Geometry check sheet. Reference: the model listing, model coordinates, mm. Face numbers are marked on the shaded views. A direction names the side the tool comes from. Give positions to 0.01 mm unless a question says otherwise; leave off trailing zeros. Loops run counter-clockwise (first coordinate to the right, second up) from the corner with the lowest first, then second, coordinate; pieces in that order, holes last. Notation, with made-up numbers: (27.25, -28.75) - (60.25, -28.75) arc R11 cw to (60.25, -18.75) - close; hole circle Ø11 at (63, 60). An arc over 180 degrees is marked (long way). Use a Markdown table: item, result. Add a question column.
1. Draft check along Z on the marked faces 3, 4 and 5. Enter one of: pulls with the +Z half, pulls with the -Z half, needs draft (parallel to the pull), parting line crosses it, or undercut.
2. Cross-section at C-C on x = -2.75. Enter the section's corners in (y, z).
3. Material ranges on L1, parallel to Z at x = 0, y = 7.75; L2, parallel to X at y = 51.5, z = 0; L3, parallel to Z at x = 3.5, y = 13, recorded low to high.
4. Cross-section at B-B on y = 35. Enter the section's corners in (x, z), and give its area (3 significant figures).
5. Cross-section at D-D on z = 4.5. Enter the section's corners in (x, y), and give its area (3 significant figures).
6. Set-up check for the marked faces 1 and 2: record each of +Z, -Z, +X, -X, +Y, -Y from which the full face is reachable in a straight line by a thin tool's end or side.
7. Cross-section at A-A on y = 5. Enter the section's corners in (x, z), and give its area (3 significant figures).
8. Depth check by flat-ended pin: P1, Ø6.5, axis at x = 0, z = 0, coming from the -Y side; P2, Ø2, axis at x = 4, y = 24.5, coming from the +Z side; P3, Ø3.5, axis at x = 0, z = 0, coming from the -Y side; P4, Ø1, axis at x = -2, y = 25.5, coming from the -Z side. Enter the tip coordinate at first touch or a pass-through.
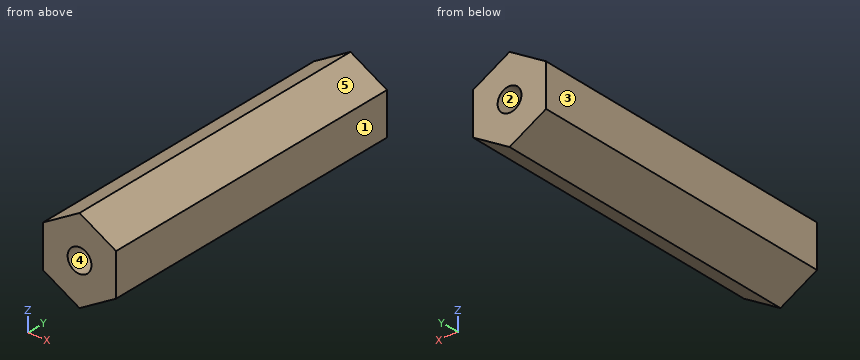
Autodesk Inventor part; units mm, degrees
ref_plane "YZ Plane" through (0, 0, 0) normal (1, 0, 0) x (0, 1, 0)
ref_plane "XZ Plane" through (0, 0, 0) normal (0, 1, 0) x (-1, 0, 0)
ref_plane "XY Plane" through (0, 0, 0) normal (0, 0, 1) x (1, 0, 0)
sketch "Sketch1" plane through (0, 0, 0) normal (0, 1, 0) x (-1, 0, 0)
  line L0 (0, 0) -> (6.35, 0)
  line L1 (6.35, -3.6662) -> (0, -7.3323)
  line L2 (0, -7.3323) -> (-6.35, -3.6662)
  line L3 (-6.35, -3.6662) -> (-6.35, 3.6662)
  line L4 (-6.35, 3.6662) -> (0, 7.3323)
  line L5 (0, 7.3323) -> (6.35, 3.6662)
  line L6 (6.35, 3.6662) -> (6.35, -3.6662)
  dimension "d0" = 6.35
extrude "Extrusion1" add sketch "Sketch1" along normal blind 58
sketch "Sketch3" plane through (0, 58, 0) normal (0, 1, 0) x (1, 0, 0)
  point P0 (0, 0)
  point P1 (0, 0)
hole "Hole1" at (0, 58, 0) direction (0, -1, 0) diameter 4.134 depth 13 tip angle 118
sketch "Sketch4" plane through (0, 0, 0) normal (0, -1, 0) x (1, 0, 0)
  point P0 (0, 0)
  point P1 (0, 0)
hole "Hole2" at (0, 0, 0) direction (0, 1, 0) diameter 4.134 depth 13 tip angle 118
properties part number "HexShaft"
Values found:
| question | item | result |
|---|---|---|
| 1 | face 3 | needs draft |
| 1 | face 4 | undercut |
| 1 | face 5 | pulls with the +Z half |
| 2 | outline | (0, -5.74) - (58, -5.74) - (58, 5.74) - (0, 5.74) - close |
| 3 | L1 | z = -7.33 to -2.07, 2.07 to 7.33 |
| 3 | L2 | x = -6.35 to -2.07, 2.07 to 6.35 |
| 3 | L3 | z = -5.31 to 5.31 |
| 4 | outline | (-6.35, -3.67) - (0, -7.33) - (6.35, -3.67) - (6.35, 3.67) - (0, 7.33) - (-6.35, 3.67) - close |
| 4 | area | 140 mm2 |
| 5 | outline | (-4.91, 0) - (4.91, 0) - (4.91, 58) - (-4.91, 58) - close |
| 5 | area | 569 mm2 |
| 6 | face 1 | +Z, -Z, +X, +Y, -Y |
| 6 | face 2 | +Y |
| 7 | outline | (-6.35, -3.67) - (0, -7.33) - (6.35, -3.67) - (6.35, 3.67) - (0, 7.33) - (-6.35, 3.67) - close; hole circle Ø4.13 at (0, 0) |
| 7 | area | 126 mm2 |
| 8 | P1 | stops at y = 0 |
| 8 | P2 | stops at z = 5.6 |
| 8 | P3 | stops at y = 13.19 |
| 8 | P4 | stops at z = -6.47 |
